Autodesk Inventor part; units mm, degrees
ref_plane "Work Plane1" through (-173.9561, 20, -439.4442) normal (0, 1, 0) x (1, 0, 0)
ref_plane "Work Plane2" through (-173.9561, 5, -439.4442) normal (0, -1, 0) x (1, 0, 0)
ref_plane "YZ Plane" through (0, 0, 0) normal (1, 0, 0) x (0, 1, 0)
sketch "Sketch1" plane through (0, 0, 0) normal (0, 1, 0) x (-1, 0, 0)
  circle A0 centre (173.9561, -439.4442) radius 14
  dimension "d17" = 28
extrude "Extrusion1" add sketch "Sketch1" against normal blind 10
sketch "Sketch2" plane through (-173.9561, -10, -439.4442) normal (0, -1, 0) x (1, 0, 0)
  circle A0 centre (0, 0) radius 15.25
  point P0 (173.9561, 439.4442)
  dimension "d20" = 30.5
extrude "Extrusion2" add sketch "Sketch2" along normal blind 12
chamfer "Chamfer1" distance 1.25 angle 45 1 edges at (-189.2061, -10, -439.4442)
sketch "Sketch4" plane through (-173.9561, -22, -439.4442) normal (0, -1, 0) x (1, 0, 0)
  circle A0 centre (0, 0) radius 14
  point P0 (173.9561, 439.4442)
  dimension "d26" = 28
extrude "Extrusion3" add sketch "Sketch4" along normal blind 0.5
sketch "Sketch5" plane through (-173.9561, -22.5, -439.4442) normal (0, -1, 0) x (1, 0, 0)
  circle A0 centre (0, 0) radius 15.25
  point P0 (173.9561, 439.4442)
  dimension "d29" = 30.5
extrude "Extrusion4" add sketch "Sketch5" along normal blind 23
sketch "Sketch6" plane through (-173.9561, -45.5, -439.4442) normal (0, -1, 0) x (1, 0, 0)
  circle A0 centre (0, 0) radius 14
  point P0 (173.9561, 439.4442)
  dimension "d32" = 28
extrude "Extrusion5" add sketch "Sketch6" along normal blind 5
sketch "Sketch7" plane through (-173.9561, 0, -439.4442) normal (0, 1, 0) x (1, 0, 0)
  circle A0 centre (0, 0) radius 15.25
  point P0 (173.9561, -439.4442)
  dimension "d35" = 30.5
extrude "Extrusion6" add sketch "Sketch7" along normal blind 30
sketch "Sketch8" plane through (-173.9561, 30, -439.4442) normal (0, 1, 0) x (1, 0, 0)
  circle A0 centre (0, 0) radius 9
  point P0 (173.9561, -439.4442)
  dimension "d38" = 18
extrude "Extrusion7" add sketch "Sketch8" along normal blind 3
sketch "Sketch10" plane through (-173.9561, 33, -439.4442) normal (0, 1, 0) x (1, 0, 0)
  circle A0 centre (0, 0) radius 6.0592
  point P0 (173.9561, -439.4442)
extrude "Extrusion9" add sketch "Sketch10" along normal blind 2
sketch "Sketch11" plane through (-173.9561, 35, -439.4442) normal (0, 1, 0) x (1, 0, 0)
  circle A0 centre (0, 0) radius 2
  point P0 (173.9561, -439.4442)
  dimension "d45" = 4
extrude "Extrusion10" add sketch "Sketch11" along normal blind 16
fillet "Fillet1" radius 0.5 1 edges at (-175.9561, 51, -439.4442)
sketch "Sketch12" plane through (-173.9561, 51, -439.4442) normal (0, 1, 0) x (1, 0, 0)
  circle A0 centre (0, 0) radius 2
  circle A1 centre (0, 0) radius 2
  line L0 (-1.75, -0.9682) -> (-1.75, 0.9682)
  line L1 (1.75, -0.9682) -> (1.75, 0.9682)
  point P0 (173.9561, -439.4442)
  dimension "d49" = 3.5
  dimension "d50" = 1.75
extrude "Extrusion11" cut sketch "Sketch12" against normal blind 14 contours A0 L1 | L0 A0
ref_plane "Work Plane1" through (-173.9561, 20, -439.4442) normal (0, 1, 0) x (1, 0, 0)
ref_plane "Work Plane2" through (-173.9561, 5, -439.4442) normal (0, -1, 0) x (1, 0, 0)
split_face "Split1"
split_face "Split2"
equation "\"d50\" = 0.5 * d49"
properties part number "14-0001"
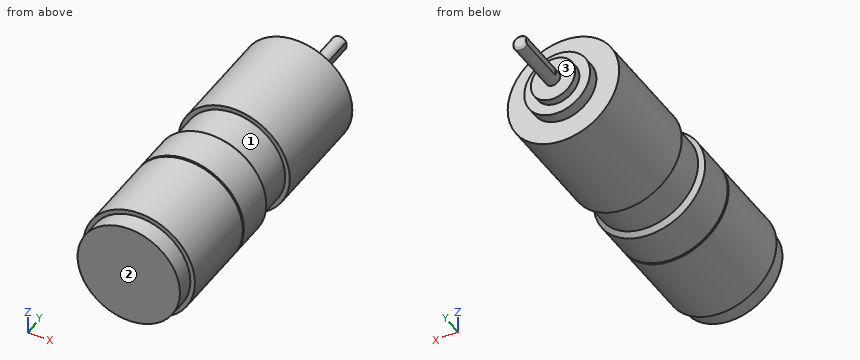
Source: CAD feature listing. Evaluate the final solid. Frame: model axes, mm. Face numbers are marked on the shaded views. A direction names the side the tool comes from. Give positions to 0.01 mm unless a question says otherwise; leave off trailing zeros. Write each loop counter-clockwise with the first axis right and the second up, starting at its lowest first coordinate (ties: lowest second). Pieces come first, ordered by that corner, then holes. Notation, with made-up numbers: (51.5, 87.25) - (69.5, 87.25) arc R33 ccw to (69.5, 117.25) - close; hole circle Ø6 at (56, 71.25). An arc over 180 degrees is marked (long way). Write item = value, one per line. Start each with the question number.
Q1. Material intervals for probe 1 along Y at (x, z) = (-172, -440); probe 2 along Y at (x, z) = (-182.5, -446); probe 3 along Y at (x, z) = (-184.5, -450), sorted ascending.
Q2. Pin query (flat end, axial travel): pin 1 Ø6 at (x, y) = (-168.5, 20.5) entering from -Z; pin 2 Ø5.5 at (x, z) = (-171, -443.5) entering from +Y; pin 3 Ø1 at (y, z) = (-8.5, -444) entering from -X; pin 4 Ø3.5 at (x, z) = (-171.5, -441) entering from +Y. Return the tip coordinate at first contact, or that it passes through.
Q3. Reachability of the marked faces 1, 2 and 3 from +Z, -Z, +X, -X, +Y, -Y: full face, straight path, thin tool, end or side. Return the list, or none.
Q4. Cut plane A-A, the plane y = -5.5. Return loops of the section in (x, z), then the cut area to 3 significant figures.
Q5. Cut plane B-B, the plane y = 16. Return loops of the section in (x, z), then the cut area to 3 significant figures.
Computed values:
q1.probe_1 = -50.5 to 35
q1.probe_2 = -50.5 to 30
q1.probe_3 = -45.5 to -22.5, -22 to -10.92, 0 to 30
q2.pin_1 = -454.5
q2.pin_2 = 35
q2.pin_3 = -187.36
q2.pin_4 = 51
q3.face_1 = none
q3.face_2 = +Z, -Z, +X, -X, -Y
q3.face_3 = +Y
q4.outline = circle Ø28 at (-173.96, -439.44)
q4.area = 616 mm²
q5.outline = circle Ø30.5 at (-173.96, -439.44)
q5.area = 731 mm²
